from build123d import *

# Parameters (mm, degrees)
SKETCH1_R           = 1.5
BOSS_EXTRUDE3_DEPTH = 3.85
BOSS_EXTRUDE4_DEPTH = 30


with BuildPart() as part:
    # Sketch1 → Boss-Extrude3 (new body, symmetric)
    with BuildSketch(Plane(origin=(0, 0, 0), x_dir=(1, 0, 0), z_dir=(0, 1, 0))):
        with BuildLine():
            Line((-13.75, -15), (0, -15))
            Line((0, -15), (0, 0))
            Line((0, 0), (2, 0))
            Line((2, 0), (2, 30))
            Line((2, 30), (-1, 30))
            ThreePointArc((-1, 30), (-1.576352013, 29.869367868), (-2.040057994, 29.503003078))
            Line((-2.040057994, 29.503003078), (-11.530466398, 17.748937838))
            ThreePointArc((-11.530466398, 17.748937838), (-13.178803317, 14.798188939), (-13.75, 11.466872681))
            Line((-13.75, 11.466872681), (-13.75, -15))
        make_face()
        with Locations((-10.75, -12)):
            Circle(SKETCH1_R, mode=Mode.SUBTRACT)
        with Locations((-3, -12)):
            Circle(SKETCH1_R, mode=Mode.SUBTRACT)
    extrude(amount=BOSS_EXTRUDE3_DEPTH, both=True)

    # Sketch2 → Boss-Extrude4 (add)
    with BuildSketch(Plane(origin=(0, 0, -30), x_dir=(-1, 0, 0), z_dir=(0, 0, -1))):
        Polygon((-2, 3.85), (-4.222798536, 0), (-2, -3.85), align=None)
    extrude(amount=-BOSS_EXTRUDE4_DEPTH)


solid = part.part
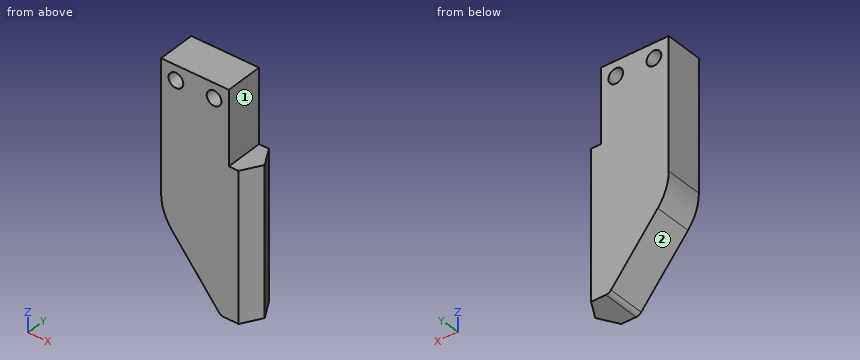
Can you work these out from the model? Positions are in its coordinate system, mm. Face numbers are marked on the shaded views. A direction names the side the tool comes from. Give positions to 0.01 mm unless a question says otherwise; leave off trailing zeros. Write each loop counter-clockwise with the first axis right and the second up, starting at its lowest first coordinate (ties: lowest second). Pieces come first, ordered by that corner, then holes. Notation, with made-up numbers: (81.5, -5.75) -> (103.5, -5.75) arc R25 ccw to (103.5, 31.25) -> close; hole circle Ø5 at (-12, 43). An arc over 180 degrees is marked (long way). Answer as a JSON object with one key per item and string values. Group by question number.
Item 1: Suppose I cut it at A-A (z = 12). Please give me the cut outline in (x, y).
Item 2: Suppose I cut it at B-B (x = -10.75). Please give me the cut outline in (y, z).
Item 3: For the marked faces 1 and 2, which set-ups out of +Z, -Z, +X, -X, +Y, -Y let a thin tool reach every point of the face, with its end or its side?
Item 4: I'm going to push flat-ended pins straight in: P1, Ø4.5, axis at x = 2.5, y = 1.5, coming from the +Z side; P2, Ø1.5, axis at y = 2, z = -6.5, coming from the +X side. Where does each tip first touch, or does it pass through?
Item 5: Suppose I cut it at C-C (y = -2). Please give me the cut outline in (x, z), plus the area to 3 significant figures.
Item 6: Please list where these lines run through material, in increasing order: line 1 (X direction, y = 2.25, z = 12); line 2 (Z direction, x = 2.5, y = 2.75); line 3 (X direction, y = 3.5, z = 8). Write a range as [from, to].
Item 7: Suppose I cut it at D-D (z = -1.5). Please give me the cut outline in (x, y), plus the area to 3 significant figures.
Findings:
{
 "1": {"outline": "(-13.75, -3.85) -> (-12.25, -3.85) -> (-12.25, 3.85) -> (-13.75, 3.85) -> close; (-9.25, -3.85) -> (-4.5, -3.85) -> (-4.5, 3.85) -> (-9.25, 3.85) -> close; (-1.5, -3.85) -> (0, -3.85) -> (0, 3.85) -> (-1.5, 3.85) -> close"},
 "2": {"outline": "(-3.85, -18.72) -> (3.85, -18.72) -> (3.85, 10.5) -> (-3.85, 10.5) -> close; (-3.85, 13.5) -> (3.85, 13.5) -> (3.85, 15) -> (-3.85, 15) -> close"},
 "3": {"face 1": "+Z, +X, +Y, -Y", "face 2": "-Z, -X, +Y, -Y"},
 "4": {"P1": "stops at z = 0", "P2": "stops at x = 3.5"},
 "5": {"outline": "(-13.75, -11.47) arc R10 ccw to (-11.53, -17.75) -> (-2.04, -29.5) arc R1.34 ccw to (-1, -30) -> (3.07, -30) -> (3.07, 0) -> (0, 0) -> (0, 15) -> (-13.75, 15) -> close; hole circle Ø3 at (-10.75, 12); hole circle Ø3 at (-3, 12)", "area": "604 mm²"},
 "6": {"line 1": "x = [-13.75, -12.25], [-9.25, -4.5], [-1.5, 0]", "line 2": "z = [-30, 0]", "line 3": "x = [-13.75, 0]"},
 "7": {"outline": "(-13.75, -3.85) -> (2, -3.85) -> (4.22, 0) -> (2, 3.85) -> (-13.75, 3.85) -> close", "area": "130 mm²"}
}
